from build123d import *

# Parameters (mm, degrees)
F2_SIZE  = 2
F3_SIZE  = 1
F4_R     = 3
F5_DEPTH = 25


with BuildPart() as f1:
    # F0 (on Front) → F1 (revolve)
    with BuildSketch(Plane.XZ):
        Polygon((57.5, 0), (32, 0), (32, -6), (35, -6), (35, -11), (32, -11), (32, -17), (35, -17), (35, -22), (32, -22), (32, -28), (40.5, -28), (40.5, -7), (57.5, -7), align=None)
    revolve(axis=Axis((0, 0, -4.022711), (0, 0, -1)))

    # F2
    f2_edges = [f1.edges().sort_by_distance(p)[0] for p in [
        (-32, 0, 0),
        (-32, 0, -28),
    ]]
    chamfer(f2_edges, length=F2_SIZE)

    # F3
    f3_edges = [f1.edges().sort_by_distance(p)[0] for p in [
        (-40.5, 0, -28),
    ]]
    chamfer(f3_edges, length=F3_SIZE)

    # F4 (on face) → F5 (cut)
    with BuildSketch(Plane.XY):
        with Locations((-36.062446, 36.062446)):
            Circle(F4_R)
        with Locations((36.062446, 36.062446)):
            Circle(F4_R)
        with Locations((36.062446, -36.062446)):
            Circle(F4_R)
        with Locations((-36.062446, -36.062446)):
            Circle(F4_R)
    extrude(amount=-F5_DEPTH, mode=Mode.SUBTRACT)


solid = f1.part
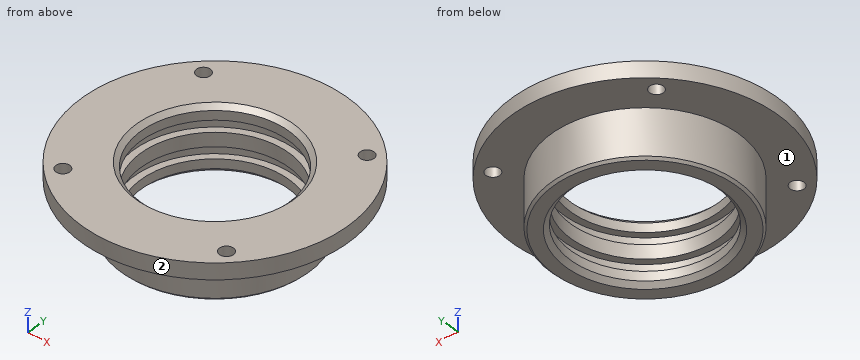
The model under review builds one solid part; all positions refer to its coordinate system, in mm. Face numbers are marked on the shaded views. A direction names the side the tool comes from. Give positions to 0.01 mm unless a question says otherwise; leave off trailing zeros. Order: outer loops, then holes, each group sorted by start corner. A loop starts at its lowest first (then second) coordinate and runs counter-clockwise, first axis right, second up. Notation, with made-up numbers: (62.25, -26) -> (93.25, -26) arc R20 cw to (93.25, 6) -> close; hole circle Ø6 at (62, -21.75). An arc over 180 degrees is marked (long way). Write item = value, one per line. Start each with the question number.
(1) Take a section at C-C (z = -20.5). Write out the cut boundary in (x, y).
(2) Tool access review of the marked faces 1 and 2: name each direction out of +Z, -Z, +X, -X, +Y, -Y from which nothing blocks a thin tool from reaching the whole face with its end or side.
(3) For pin 1 Ø1 at (x, y) = (-34.5, -23) entering from -Z; pin 2 Ø3 at (y, z) = (-8.5, -17) entering from -X; pin 3 Ø10 at (y, z) = (-16.5, -15) entering from +X, all flat-tipped, find the tip position at first contact; note any pin that passes through.
(4) For L1, parallel to X at y = 0, z = -24; L2, parallel to Y at x = 0, z = -9.85; L3, parallel to Y at x = 0, z = -2.75, list the stretches that pass through material, from the lowest coordinate up. Write a range as from..to.
(5) Take a section at D-D (y = -45.5). Write out the cut boundary in (x, z).
Returned:
q1.outline = circle Ø81 at (0, 0); hole circle Ø70 at (0, 0)
q2.face_1 = -Z
q2.face_2 = +Z, -Z
q3.pin_1 = -7
q3.pin_2 = -39.89
q3.pin_3 = 38.83
q4.L1 = -40.5..-32, 32..40.5
q4.L2 = -40.5..-35, 35..40.5
q4.L3 = -57.5..-32, 32..57.5
q5.outline = (-35.16, -7) -> (35.16, -7) -> (35.16, 0) -> (-35.16, 0) -> close
